Geometry: final body of the model. Coordinates: model frame, mm. A direction names the side the tool comes from. Coordinates: 2 decimals unless noted, no trailing zeros. Order: outer loops, then holes, each group sorted by start corner. A loop starts at its lowest first (then second) coordinate and runs counter-clockwise, first axis right, second up. Notation, with made-up numbers: (62, 38) -> (72, 38) arc R25 cw to (72, 63) -> close; hole circle Ø7 at (20.25, 9.25). An arc over 180 degrees is marked (long way). Use one line per item in the form item = value.
```python
from build123d import *

# Parameters (mm, degrees)
SKETCH1_R      = 14.1
EXTRUDE1_DEPTH = 15.5
SKETCH2_R      = 11.5
EXTRUDE2_DEPTH = 5
CHAMFER1_SIZE  = 0.5
SKETCH3_R      = 11.617958336
EXTRUDE3_DEPTH = 3


with BuildPart() as part:
    # Sketch1 → Extrude1 (new body)
    with BuildSketch(Plane(origin=(0, 0, 0), x_dir=(1, 0, 0), z_dir=(0, 1, 0))):
        with Locations(Location((0, 0, 0), (0, 0, 270))):
            Circle(SKETCH1_R)
    extrude(amount=EXTRUDE1_DEPTH)

    # Sketch2 → Extrude2 (add)
    with BuildSketch(Plane(origin=(0, 15.5, 0), x_dir=(1, 0, 0), z_dir=(0, 1, 0))):
        with Locations(Location((0, 0, 0), (0, 0, 270))):
            Circle(SKETCH2_R)
    extrude(amount=EXTRUDE2_DEPTH)

    # Chamfer1
    chamfer1_edges = [part.edges().sort_by_distance(p)[0] for p in [
        (0, 20.5, -11.5),
    ]]
    chamfer(chamfer1_edges, length=CHAMFER1_SIZE)

    # Sketch3 → Extrude3 (cut)
    with BuildSketch(Plane.XZ):
        with Locations(Location((0, 0, 0), (0, 0, 270))):
            Circle(SKETCH3_R)
    extrude(amount=-EXTRUDE3_DEPTH, mode=Mode.SUBTRACT)


solid = part.part
```
1) Contact query for flat-ended pins moving along their axis: P1, Ø1, axis at y = 11, z = -4, coming from the +X side; P2, Ø3, axis at y = 3, z = -5, coming from the -X side; P3, Ø2, axis at y = 7.5, z = -2.5, coming from the +X side; P4, Ø3, axis at y = 9.5, z = -0.5, coming from the +X side. Output: stop coordinate, or through.
Results found:
P1 = 13.66
P2 = -13.66
P3 = 14.02
P4 = 14.1
2) Pull-direction query (Z, two-part tool) for faces 4 (the cylindrical face through (9.7, 17.72, 6.18)), 5 (the flat face through (12, 0, 2)), 6 (the flat face through (0, 3, 0)); classes: released by +Z, released by -Z, zero draft, split by the parting line, or undercut.
Results found:
face_4 = split by the parting line
face_5 = zero draft
face_6 = undercut
3) Section B-B, the plane x = 0. Output: boundary loops of the cut face in (y, z), and give its area (3 significant figures).
Results found:
outline = (0, -14.1) -> (15.5, -14.1) -> (15.5, -11.5) -> (20, -11.5) -> (20.5, -11) -> (20.5, 11) -> (20, 11.5) -> (15.5, 11.5) -> (15.5, 14.1) -> (0, 14.1) -> (0, 11.62) -> (3, 11.62) -> (3, -11.62) -> (0, -11.62) -> close
area = 482 mm2
4) Access query for faces 1 (the flat face through (0, 20.5, 0)), 2 (the cylindrical face through (3.49, 1.48, -11.08)), 3 (the flat face through (0, 15.5, -12)). Directions: +Z, -Z, +X, -X, +Y, -Y. A direction counts if a zero-diameter tool reaches every point of the face in a straight line with its end or side. Return the directions, or none.
Results found:
face_1 = +Z, -Z, +X, -X, +Y
face_2 = -Y
face_3 = +Y
5) Section C-C, the plane y = 12.5. Output: boundary loops of the cut face in (x, z).
Results found:
outline = circle Ø28.2 at (0, 0)
6) Material intervals for probe 1 along X at (y, z) = (0.8, 0); probe 2 along Y at (x, z) = (-8, 7.25); probe 3 along Z at (x, y) = (0.25, 18.25), sorted ascending. Write a range as from..to.
Results found:
probe_1 = -14.1..-11.62, 11.62..14.1
probe_2 = 3..20.5
probe_3 = -11.5..11.5
7) Section D-D, the plane y = 17. Output: boundary loops of the cut face in (x, z).
Results found:
outline = circle Ø23 at (0, 0)
8) Section A-A, the plane z = 0. Output: boundary loops of the cut face in (x, y).
Results found:
outline = (-14.1, 0) -> (-11.62, 0) -> (-11.62, 3) -> (11.62, 3) -> (11.62, 0) -> (14.1, 0) -> (14.1, 15.5) -> (11.5, 15.5) -> (11.5, 20) -> (11, 20.5) -> (-11, 20.5) -> (-11.5, 20) -> (-11.5, 15.5) -> (-14.1, 15.5) -> close
